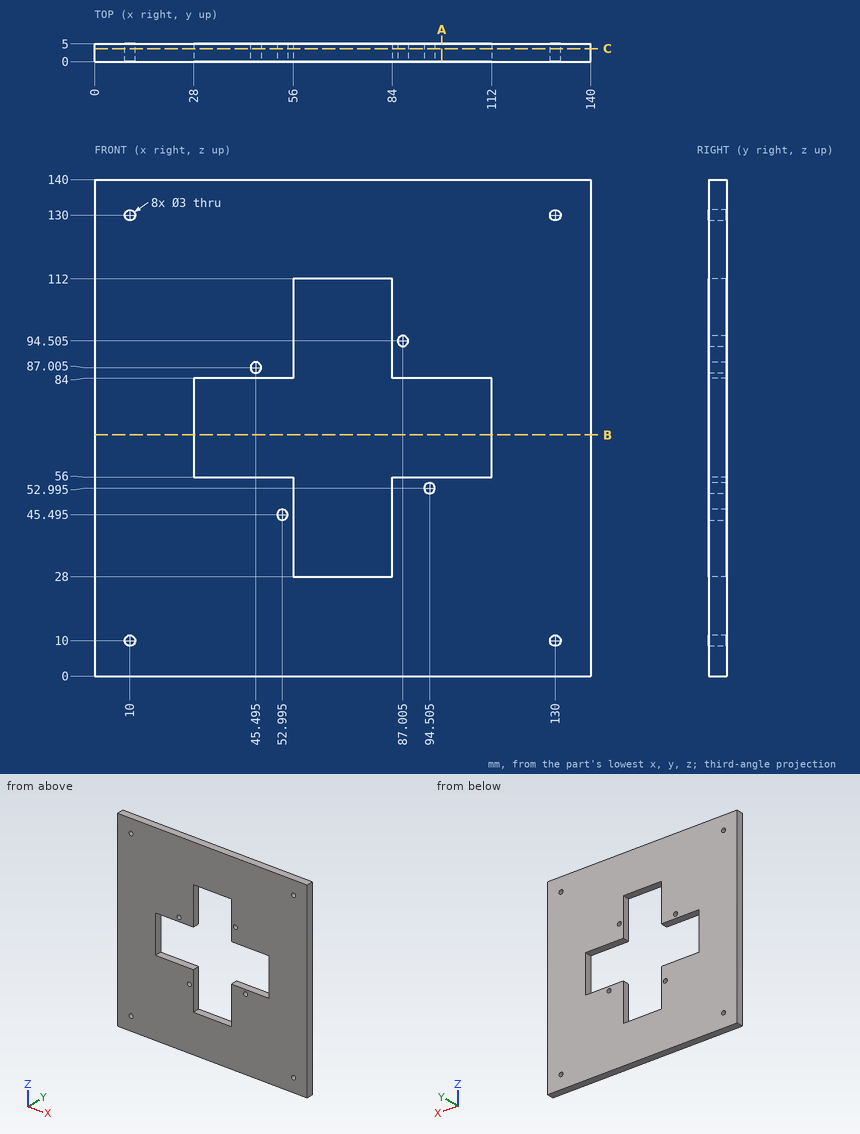
The figure shows three views and two pictorial views of one solid part (mm, origin at its lowest corner). Answer the questions. Coordinates: 2 decimals unless noted, no trailing zeros. Write each loop counter-clockwise with the first axis right and the second up, starting at its lowest first coordinate (ties: lowest second). Pieces come first, ordered by that corner, then holes. Notation, with made-up numbers: (18, -12) -> (73, -12) arc R30 ccw to (73, 26) -> close; hole circle Ø4 at (0, 67). An arc over 180 degrees is marked (long way). Return JSON: item names as keys, results as strings.
1. Each of these flat-tipped pins is pushed along its axis until it touches: P1, Ø2.5, axis at x = 76.5, y = 2, coming from the -Z side; P2, Ø1.8, axis at x = 94.505, z = 52.995, coming from the -Y side. Where does it stop, or does it pass through?
Found:
{"P1": "z = 0", "P2": "through"}
2. Find the intervals of material crossed by line 1 along Z through (x, y) = (10, 3.8); line 2 along Z through (x, y) = (91, 3.05), in increasing order. Write a range as from..to.
Found:
{"line 1": "0..8.5, 11.5..128.5, 131.5..140", "line 2": "0..56, 84..140"}
3. A cutting plane is placed at B-B (z = 68). Determine the outline of the cut face in (x, y), and give its area (3 significant figures).
Found:
{"outline": "(0, 0) -> (28, 0) -> (28, 5) -> (0, 5) -> close; (112, 0) -> (140, 0) -> (140, 5) -> (112, 5) -> close", "area": "280 mm2"}
4. A cutting plane is placed at C-C (y = 3.7). Give the number of separate pieces and of enclosed holes in the cut face, and give its area (3 significant figures).
Found:
{"separate pieces": "1", "enclosed holes": "9", "area": "15,600 mm2"}
5. A cutting plane is placed at A-A (x = 98). Determine the outline of the cut face in (y, z).
Found:
{"outline": "(0, 0) -> (5, 0) -> (5, 56) -> (0, 56) -> close; (0, 84) -> (5, 84) -> (5, 140) -> (0, 140) -> close"}
